Autodesk Inventor part; units mm, degrees
ref_plane "YZ Plane" through (0, 0, 0) normal (1, 0, 0) x (0, 1, 0)
ref_plane "XZ Plane" through (0, 0, 0) normal (0, 1, 0) x (-1, 0, 0)
ref_plane "XY Plane" through (0, 0, 0) normal (0, 0, 1) x (1, 0, 0)
sketch "Szkic1" plane through (0, 0, 0) normal (0, 0, 1) x (1, 0, 0)
  circle A0 centre (0.2713, 9.4144) radius 2
  circle A1 centre (0.2713, -9.4144) radius 2
  ellipse E0 centre (-8.3642, 0) end of major axis (-1.8423, 0) minor radius 6 (-14.886, 0) -> (-13.7374, -3.4005) ccw
  spline S0 degree 3 poles (-3.8083, -16.5118) (-7.4967, -13.768) (-11.3809, -9.2364) (-13.7374, -3.4005) knots 1 1 1 1 1.842723 1.842723 1.842723 1.842723
  line L0 (7.3687, -16.5118) -> (-3.8083, -16.5118)
  spline S1 degree 3 poles (4.6424, 0) (7.5886, -2.9462) (10.6572, -15.0638) (7.3687, -16.5118) knots 1 1 1 1 2 2 2 2
  spline S2 degree 3 poles (7.3687, 16.5118) (10.6572, 15.0638) (7.5886, 2.9462) (4.6424, 0) knots 1 1 1 1 2 2 2 2
  line L1 (-3.8083, 16.5118) -> (7.3687, 16.5118)
  spline S3 degree 3 poles (-13.7374, 3.4005) (-11.3809, 9.2364) (-7.4967, 13.768) (-3.8083, 16.5118) knots 1.157277 1.157277 1.157277 1.157277 2 2 2 2
  ellipse E1 centre (-8.3642, 0) end of major axis (-1.8423, 0) minor radius 6 (-13.7374, 3.4005) -> (-14.886, 0) ccw
  ellipse E2 centre (-7.9381, 0) end of major axis (-1.4162, 0) minor radius 6
  point P0 (0, 0)
extrude "Wyciągnięcie proste1" add sketch "Szkic1" along normal blind 1
properties part number "mocowanie_podwozia_gora"
For this review, take the finished solid that the model builds, in its own axes (mm). Round coordinates to 2 decimals unless told otherwise and drop trailing zeros. One line per question, with ' | ' between items.
Q1. The part is to be moulded in two halves that separate along X. For faces 1 (the cylindrical face through (0.01, 7.43, 0.49)), 2 (the flat face through (1, 0, 1)), say which applies: released by +X, released by -X, zero draft, split by the parting line, or undercut.
Taken from the geometry:
face 1: undercut | face 2: zero draft
Q2. For line 1 along Y through (x, z) = (1.5, 0.75); line 2 along Y through (x, z) = (-9.75, 0.2); line 3 along Y through (x, z) = (-0.5, 0.8), list the stretches that pass through material, from the lowest coordinate up. Write a range as [from, to].
Taken from the geometry:
line 1: y = [-16.51, -10.99], [-7.84, 7.84], [10.99, 16.51] | line 2: y = [-10.49, -5.76], [5.76, 10.49] | line 3: y = [-16.51, -11.26], [-7.57, 7.57], [11.26, 16.51]
Q3. Take a section at A-A (z = 0.75). State how many separate pieces and enclosed holes the cut face has, and give its area (3 significant figures).
Taken from the geometry:
separate pieces: 1 | enclosed holes: 3 | area: 459 mm²
